```python
from build123d import *

# Parameters (mm, degrees)
F0_R = 15


with BuildPart() as f3:
    # F3: sweep along a path in F2
    with BuildLine(Plane.XZ.offset(36.91316396)) as f3_path:
        Line((-399.0737497807, 0), (-399.0737497807, -765))
        ThreePointArc((-399.0737497807, -765), (-393.2158854044, -779.1421356237), (-379.0737497807, -785))
        Line((-379.0737497807, -785), (480.9262502193, -785))
        ThreePointArc((480.9262502193, -785), (495.0683858431, -779.1421356237), (500.9262502193, -765))
        Line((500.9262502193, -765), (500.9262502193, 0))
    # F0 (on Top) → F3 (sweep)
    with BuildSketch(Plane.XY):
        with Locations((-399.0737497807, -36.91316396)):
            Circle(F0_R)
    sweep(path=f3_path.line)


solid = f3.part
```
The model under review builds one solid part; all positions refer to its coordinate system, in mm. A direction names the side the tool comes from. Coordinates: 2 decimals unless noted, no trailing zeros. Write each loop counter-clockwise with the first axis right and the second up, starting at its lowest first coordinate (ties: lowest second). Pieces come first, ordered by that corner, then holes. Notation, with made-up numbers: (12, 28) - (41, 28) arc R13 ccw to (41, 50) - close; hole circle Ø1 at (-39.5, 63). An arc over 180 degrees is marked (long way). Answer in a Markdown table with one row per item. Add a question column.
Q1. To check wall thickness, follow line 1 along X through (y, z) = (-39, -168); line 2 along X through (y, z) = (-37.5, -525.5); line 3 along Z through (x, y) = (32.5, -38.5). State the ranges of each line that lie inside material, in increasing order. Write a range as from..to.
Q2. For faces 3 (the face through (515.91, -37.57, -377.14)), 4 (the face through (501, -37, 0)), list the 3-axis set-ups (+Z, -Z, +X, -X, +Y, -Y) from which the entire face can be reached by the end or side of a thin tool; tool diameter is ignored.
Q3. Consider section B-B on z = -733. Give the boundary of the cut face in (x, y).
Q4. Consider section A-A on y = -31. Give the boundary of the cut face in (x, z), then the cut area to 3 significant figures.
Q5. Clearance check with flat-ended pins moving along their axes: pin 1 (1.5 mm diameter, centred on y = -39.5, z = -717, fed in from +X); pin 2 (2 mm diameter, centred on x = -270.5, y = -30.5, fed in from -Z); pin 3 (10 mm diameter, centred on x = -108.5, y = -42.5, fed in from +Z). State where each tip first meets the part, or that it passes through.
Q6. Consider section C-C on x = -77.5. Give the boundary of the cut face in (y, z), then the cut area to 3 significant figures.
Q7. Draft analysis for pull direction X (two halves, no side actions). For faces 1 (the face through (-399, -37, 0)), 2 (the face through (56.946, -31.168, -771.144)), state which applies: +X half, -X half, draft (parallel to the pull), parting line (faces both ways), or undercut.
Answers below:
| question | item | result |
|---|---|---|
| 1 | line 1 | -413.93..-384.22, 486.07..515.78 |
| 1 | line 2 | -414.06..-384.09, 485.94..515.91 |
| 1 | line 3 | -799.92..-770.08 |
| 2 | face 3 | +Z |
| 2 | face 4 | +Z, +X, -X, +Y, -Y |
| 3 | outline | circle Ø30 at (-399.07, -36.91); circle Ø30 at (500.93, -36.91) |
| 4 | outline | (-412.86, -765) arc R33.79 ccw to (-379.07, -798.79) - (480.93, -798.79) arc R33.79 ccw to (514.71, -765) - (514.71, 0) - (487.14, 0) - (487.14, -765) arc R6.21 cw to (480.93, -771.21) - (-379.07, -771.21) arc R6.21 cw to (-385.29, -765) - (-385.29, 0) - (-412.86, 0) - close |
| 4 | area | 67,600 mm² |
| 5 | pin 1 | x = 515.81 |
| 5 | pin 2 | z = -798.99 |
| 5 | pin 3 | z = -770.01 |
| 6 | outline | circle Ø30 at (-36.91, -785) |
| 6 | area | 707 mm² |
| 7 | face 1 | draft |
| 7 | face 2 | undercut |
